Input: part model. Units: mm. Frame: model coordinates. A direction names the side the tool comes from. Round coordinates to 2 decimals unless told otherwise and drop trailing zeros. Loops run counter-clockwise (first coordinate to the right, second up) from the corner with the lowest first, then second, coordinate; pieces in that order, holes last. Notation, with made-up numbers: M 17.5,26.5 L 46.5,26.5 A7 cw 46.5,35.5 Z; hole C 51,85.25 d9. An arc over 180 degrees is marked long. Return JSON: item names as keys, results as strings. Group by question number.
1) Contact query for flat-ended pins moving along their axis: P1, Ø5, axis at y = -0.5, z = 8.5, coming from the +X side; P2, Ø10, axis at x = 6, z = 6, coming from the +Y side; P3, Ø5, axis at y = -7, z = 12, coming from the +X side; P4, Ø4, axis at y = 40.5, z = 6.5, coming from the -X side. Output: stop coordinate, or through.
2) Section D-D (z = 17.5). Output: boundary loops of the cut face in (x, y), plus the area to 4 significant figures.
3) Mould query, pull axis Y, two halves, no side actions, for faces 5 (the face through (6, -43, 5)), 6 (the face through (2, 32.75, 10)), 7 (the face through (5, -46, 5)). Classes: +Y half, -Y half, draft (parallel to the pull), parting line (faces both ways), or undercut.
4) Material intervals for line 1 (Y direction, x = 11.5, z = 4.25); line 2 (X direction, y = -29.5, z = 15.5), sorted ascending. Write a range as from..to.
5) Section A-A (z = 10). Count the separate pieces of the cut face and the enclosed holes in it, plus the area to 3 significant figures.
6) Section B-B (x = 9.75). Output: boundary loops of the cut face in (y, z), plus the area to 3 significant figures.
7) Access query for faces 1 (the face through (4, -31, 4)), 2 (the face through (8, -40.56, 8)), 3 (the face through (8, 2.5, 8)), 4 (the face through (0, 39, 10)). Directions: +Z, -Z, +X, -X, +Y, -Y. A direction counts if a zero-diameter tool reaches every point of the face in a straight line with its end or side. Return the directions, or none.
8) Section C-C (y = 13). Output: boundary loops of the cut face in (x, z), plus the area to 4 significant figures.
from build123d import *

# Parameters (mm, degrees)
F1_DEPTH  = 46
F2_SIZE   = 5
F6_DEPTH  = 2.5
F8_DEPTH  = 2.5
F10_DEPTH = 2.5
F11_W     = 4
F11_H     = 3
F12_DEPTH = 20.001
F15_DEPTH = 5
F18_DEPTH = 5
F19_W     = 59.5
F19_H     = 20
F20_DEPTH = 7


with BuildPart() as f1:
    # F0 (on Front) → F1 (new body, symmetric)
    with BuildSketch(Plane.XZ):
        Polygon((0, 20), (0, 0), (20, 0), (20, 3), (3, 3), (3, 20), align=None)
    extrude(amount=F1_DEPTH, both=True)

    # F2
    f2_edges = [f1.edges().sort_by_distance(p)[0] for p in [
        (3, 0, 3),
    ]]
    chamfer(f2_edges, length=F2_SIZE)

    # F5 (on Front) → F6 (join, symmetric)
    with BuildSketch(Plane.XZ):
        Polygon((15.7, 3), (3, 15.7), (3, 3), align=None)
    extrude(amount=F6_DEPTH, both=True)

    # F7 (on offset) → F8 (join, symmetric)
    with BuildSketch(Plane.XZ.offset(19.05)):
        Polygon((15.7, 3), (3, 15.7), (3, 3), align=None)
    extrude(amount=F8_DEPTH, both=True)

    # F9 (on offset) → F10 (join, symmetric)
    with BuildSketch(Plane.XZ.offset(-19.05)):
        Polygon((15.7, 3), (3, 15.7), (3, 3), align=None)
    extrude(amount=F10_DEPTH, both=True)

    # F11 (on face) → F12 (cut, through all)
    with BuildSketch(Plane.XY.offset(20)):
        with Locations((2, 31.25)):
            Rectangle(F11_W, F11_H)
        with Locations((2, -31.25)):
            Rectangle(F11_W, F11_H)
    extrude(amount=-F12_DEPTH, mode=Mode.SUBTRACT)

    # F14 (on offset) → F15 (join)
    with BuildSketch(Plane.XZ.offset(35.56)):
        Polygon((8, 3), (15.7, 3), (3, 15.7), (3, 8), align=None)
    extrude(amount=F15_DEPTH)

    # F17 (on offset) → F18 (join)
    with BuildSketch(Plane.XZ.offset(-35.56)):
        Polygon((15.7, 3), (3, 15.7), (3, 8), (8, 3), align=None)
    extrude(amount=-F18_DEPTH)

    # F19 (on face) → F20 (join)
    with BuildSketch(Plane(origin=(0, 0, 0), x_dir=(0, -1, 0), z_dir=(-1, 0, 0))):
        with Locations((0, 10)):
            Rectangle(F19_W, F19_H)
    extrude(amount=F20_DEPTH)


solid = f1.part
Returned:
{
 "1": {"P1": "stops at x = 12.7", "P2": "stops at y = 46", "P3": "stops at x = 3", "P4": "stops at x = 0"},
 "2": {"outline": "M -7,-29.75 L 3,-29.75 L 3,29.75 L -7,29.75 Z; M 0,-46 L 3,-46 L 3,-32.75 L 0,-32.75 Z; M 0,32.75 L 3,32.75 L 3,46 L 0,46 Z", "area": "674.5 mm^2"},
 "3": {"face 5": "draft", "face 6": "undercut", "face 7": "-Y half"},
 "4": {"line 1": "y = -40.56..-35.56, -21.55..-16.55, -2.5..2.5, 16.55..21.55, 35.56..40.56", "line 2": "x = -7..3"},
 "5": {"separate pieces": "3", "enclosed holes": "0", "area": "817 mm^2"},
 "6": {"outline": "M -46,0 L 46,0 L 46,3 L 40.56,3 L 40.56,8.95 L 35.56,8.95 L 35.56,3 L 21.55,3 L 21.55,8.95 L 16.55,8.95 L 16.55,3 L 2.5,3 L 2.5,8.95 L -2.5,8.95 L -2.5,3 L -16.55,3 L -16.55,8.95 L -21.55,8.95 L -21.55,3 L -35.56,3 L -35.56,8.95 L -40.56,8.95 L -40.56,3 L -46,3 Z", "area": "425 mm^2"},
 "7": {"face 1": "+Z, -Z, -X", "face 2": "+Z, +X, -Y", "face 3": "+Z, +X", "face 4": "+Z, -Z, -X, +Y"},
 "8": {"outline": "M -7,0 L 20,0 L 20,3 L 8,3 L 3,8 L 3,20 L -7,20 Z", "area": "263.5 mm^2"}
}
